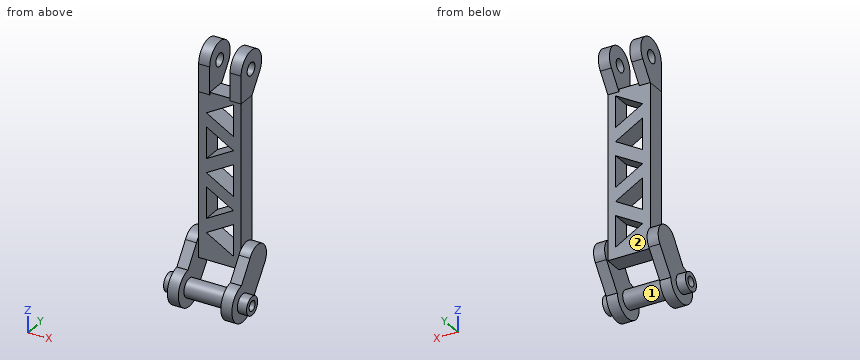
from build123d import *

# Parameters (mm, degrees)
SKETCH023_R       = 3.5
EXTRUDE022_DEPTH  = 6
SKETCH021_W       = 23
SKETCH021_H       = 90
EXTRUDE020_DEPTH  = 10
CYLINDER028_R     = 3
CYLINDER028_DEPTH = 25
CYLINDER027_R     = 7
CYLINDER027_DEPTH = 30
CYLINDER026_R     = 10
CYLINDER026_DEPTH = 6
EXTRUDE021_DEPTH  = 6
CYLINDER030_R     = 2.7
CYLINDER030_DEPTH = 50
CYLINDER029_R     = 5
CYLINDER029_DEPTH = 45


with BuildPart() as union_brazo_central004:
    # Sketch023 → Extrude022 (new body)
    with BuildSketch(Plane(origin=(0, 0, 0), x_dir=(0, -1, 0), z_dir=(-1, 0, 0))):
        with BuildLine():
            ThreePointArc((-10.966848, 145.524062), (-23.171274, 154.396494), (-27.829317, 140.044816))
            Line((-27.829317, 140.044816), (-20.975712, 130.624062))
            Line((-20.975712, 130.624062), (-10.975712, 130.624062))
            Line((-10.966848, 145.524062), (-10.975712, 130.624062))
        make_face()
        with Locations((-20.000471, 144.992747)):
            Circle(SKETCH023_R, mode=Mode.SUBTRACT)
    extrude(amount=EXTRUDE022_DEPTH)


with BuildPart() as union_brazo_central004_1:
    # Extrude022 placement: moved
    add(union_brazo_central004.part.moved(Location((62.99, 0, 0))))


with BuildPart() as union_brazo_central005:
    # Link021 base: copy of Union brazo central004
    add(union_brazo_central004_1.part)


with BuildPart() as union_brazo_central005_1:
    # Link021 placement: moved
    add(union_brazo_central005.part.moved(Location((17.001, 0, 0))))


with BuildPart() as obj1:
    # Sketch021 → Extrude020 (new body)
    with BuildSketch(Plane.XZ):
        with Locations((68.040845, 88.110787)):
            Rectangle(SKETCH021_W, SKETCH021_H)
        Polygon((60.680845, 57.610787), (75.403277, 66.110787), (75.403277, 49.110787), align=None, mode=Mode.SUBTRACT)
        Polygon((60.678413, 65.110787), (60.678413, 82.110787), (75.400845, 73.610787), align=None, mode=Mode.SUBTRACT)
        Polygon((60.680845, 89.610787), (75.403277, 98.110787), (75.403277, 81.110787), align=None, mode=Mode.SUBTRACT)
        Polygon((60.678413, 97.110787), (60.678413, 114.110787), (75.400845, 105.610787), align=None, mode=Mode.SUBTRACT)
        Polygon((60.680845, 121.610787), (75.403277, 130.110787), (75.403277, 113.110787), align=None, mode=Mode.SUBTRACT)
    extrude(amount=EXTRUDE020_DEPTH)


with BuildPart() as obj1_1:
    # Extrude020 placement: moved
    add(obj1.part.moved(Location((0.45, 21, -1.11))))


with BuildPart() as rotor011:
    # Cylinder028 → Cylinder028 (new body)
    with BuildSketch(Plane(origin=(40, 2.5, 30), x_dir=(0, 0, -1), z_dir=(1, 0, 0))):
        Circle(CYLINDER028_R)
    extrude(amount=CYLINDER028_DEPTH)


with BuildPart() as rotor010:
    # Cylinder027 → Cylinder027 (new body)
    with BuildSketch(Plane(origin=(63, 2.5, 30), x_dir=(0, 0, -1), z_dir=(1, 0, 0))):
        Circle(CYLINDER027_R)
    extrude(amount=CYLINDER027_DEPTH)


with BuildPart() as obj2:
    # Cylinder026 → Cylinder026 (new body)
    with BuildSketch(Plane(origin=(54, 2.5, 30), x_dir=(0, 0, -1), z_dir=(1, 0, 0))):
        Circle(CYLINDER026_R)
    extrude(amount=CYLINDER026_DEPTH)

    # Cut013: cut Rotor010
    add(rotor010.part, mode=Mode.SUBTRACT)

    # Cut014: cut Rotor011
    add(rotor011.part, mode=Mode.SUBTRACT)


with BuildPart() as union_motor_centro002:
    # Sketch022 → Extrude021 (new body)
    with BuildSketch(Plane.YZ):
        with BuildLine():
            ThreePointArc((22.654639, 41.99706), (20.679007, 53.483206), (9.335322, 50.808228))
            Line((9.335322, 50.808228), (1.552816, 39.899855))
            ThreePointArc((12.665635, 28.738862), (9.310536, 36.511168), (1.552816, 39.899855))
            Line((22.654639, 41.99706), (12.665635, 28.738862))
        make_face()
    extrude(amount=EXTRUDE021_DEPTH)


with BuildPart() as union_motor_centro002_1:
    # Extrude021 placement: moved
    add(union_motor_centro002.part.moved(Location((54, -0.35, 0))))

    # Fusion024: union obj2
    add(obj2.part)


with BuildPart() as union_motor_centro003:
    # Link020 base: copy of Union motor centro002
    add(union_motor_centro002_1.part)


with BuildPart() as union_motor_centro003_1:
    # Link020 placement: moved
    add(union_motor_centro003.part.moved(Location((28.999998, -3e-06, 0))))


with BuildPart() as hueco_rotor001:
    # Cylinder030 → Cylinder030 (new body)
    with BuildSketch(Plane(origin=(37, 2.5, 30), x_dir=(0, 0, -1), z_dir=(1, 0, 0))):
        Circle(CYLINDER030_R)
    extrude(amount=CYLINDER030_DEPTH)


with BuildPart() as brazo_central_v3:
    # Cylinder029 → Cylinder029 (new body)
    with BuildSketch(Plane(origin=(40, 2.5, 30), x_dir=(0, 0, -1), z_dir=(1, 0, 0))):
        Circle(CYLINDER029_R)
    extrude(amount=CYLINDER029_DEPTH)

    # Cut015: cut hueco rotor001
    add(hueco_rotor001.part, mode=Mode.SUBTRACT)


with BuildPart() as brazo_central_v3_1:
    # Cut015 placement: moved
    add(brazo_central_v3.part.moved(Location((9, 0, 0))))

    # Fusion025: union Union motor centro003, Union motor centro002
    add(union_motor_centro003_1.part)
    add(union_motor_centro002_1.part)


with BuildPart() as brazo_central_v3_2:
    # Fusion025 placement: moved
    add(brazo_central_v3_1.part.moved(Location((-3, 0, 0))))

    # Fusion026: union Union brazo central004, Union brazo central005, obj1
    add(union_brazo_central004_1.part)
    add(union_brazo_central005_1.part)
    add(obj1_1.part)


solid = brazo_central_v3_2.part
Can you work these out from the model? Positions are in its coordinate system, mm. Face numbers are marked on the shaded views. A direction names the side the tool comes from. Give positions to 0.01 mm unless a question says otherwise; leave off trailing zeros. Loops run counter-clockwise (first coordinate to the right, second up) from the corner with the lowest first, then second, coordinate; pieces in that order, holes last. Notation, with made-up numbers: (-24, 25.25) -> (20, 25.25) arc R16 ccw to (20, 41.25) -> close; hole circle Ø5 at (12, -6.5). An arc over 180 degrees is marked (long way). Return JSON: item names as keys, results as strings.
Q1. I want a section at D-D, the plane x = 88.5. List the corners of the cut face in (y, z) for me, then the cut area to 3 significant figures.
Checks:
{"outline": "circle Ø10 at (2.5, 30); hole circle Ø5.4 at (2.5, 30)", "area": "55.6 mm2"}
Q2. I want a section at B-B, the plane x = 72.5. List the corners of the cut face in (y, z) for me, then the cut area to 3 significant figures.
Checks:
{"outline": "circle Ø10 at (2.5, 30); (11, 42) -> (21, 42) -> (21, 49.94) -> (11, 49.94) -> close; (11, 63.06) -> (21, 63.06) -> (21, 70.57) -> (11, 70.57) -> close; (11, 74.44) -> (21, 74.44) -> (21, 81.94) -> (11, 81.94) -> close; (11, 95.06) -> (21, 95.06) -> (21, 102.57) -> (11, 102.57) -> close; (11, 106.44) -> (21, 106.44) -> (21, 113.94) -> (11, 113.94) -> close; (11, 127.06) -> (21, 127.06) -> (21, 132) -> (11, 132) -> close; hole circle Ø5.4 at (2.5, 30)", "area": "484 mm2"}
Q3. I want a section at C-C, the plane y = 4. List the corners of the cut face in (x, z) for me (3 decimals), then the cut area to 3 significant figures.
Checks:
{"outline": "(46, 25.23) -> (51, 25.23) -> (51, 20.113) -> (57, 20.113) -> (57, 25.23) -> (80, 25.23) -> (80, 20.113) -> (86, 20.113) -> (86, 25.23) -> (91, 25.23) -> (91, 27.755) -> (46, 27.755) -> close; (46, 32.245) -> (91, 32.245) -> (91, 34.77) -> (86, 34.77) -> (86, 43.821) -> (80, 43.821) -> (80, 34.77) -> (57, 34.77) -> (57, 43.821) -> (51, 43.821) -> (51, 34.77) -> (46, 34.77) -> close", "area": "397 mm2"}
Q4. For pin 1 Ø15 at (y, z) = (19.5, 140) entering from +X; pin 2 Ø3 at (x, y) = (66, 14) entering from +Z; pin 3 Ø4 at (x, z) = (79, 103) entering from +Y, each with a flat end and sliding along its axis, tell me the tip position at first contact or that it passes through.
Checks:
{"pin 1": "stops at x = 79.99", "pin 2": "stops at z = 132", "pin 3": "stops at y = 21"}
Q5. I want a section at A-A, the plane z = 99. List the corners of the cut face in (x, y) for me.
Checks:
{"outline": "(56.99, 11) -> (61.13, 11) -> (61.13, 21) -> (56.99, 21) -> close; (66.32, 11) -> (79.99, 11) -> (79.99, 21) -> (66.32, 21) -> close"}
Q6. On a 3-axis mill with a long thin cutter (end or side, diameter ignored), from which of +Z, -Z, +X, -X, +Y, -Y can I reach the whole of each face in a straight line? I mean the marked faces 1 and 2. Say none if no direction works.
Checks:
{"face 1": "none", "face 2": "-Z, +Y"}
Q7. I need wall thicknesses on probe 1 along Y at (x, z) = (79, 44.5); probe 2 along Z at (x, y) = (72, 20.5); probe 3 along X at (y, z) = (26, 147). Which ranges of each line are inside material? Lowest first, please.
Checks:
{"probe 1": "y = 11 to 21", "probe 2": "z = 42 to 50.23, 62.78 to 70.28, 74.72 to 82.23, 94.78 to 102.28, 106.72 to 114.23, 126.78 to 132", "probe 3": "x = 56.99 to 62.99, 73.99 to 79.99"}
